from build123d import *

# Parameters (mm, degrees)
SKETCH_1_W          = 76
SKETCH_1_H          = 60
EXTRUDE_3_DEPTH     = 5.8
SKETCH_4_R          = 5.1
SKETCH_4_R_2        = 1.6
CUT_EXTRUDE_2_DEPTH = 50
FILLET_4_R          = 5
CUT_EXTRUDE_7_DEPTH = 13.5
FILLET_8_R          = 5
SKETCH_11_R         = 1
CUT_EXTRUDE_8_DEPTH = 49.76105003
SKETCH_12_R         = 1.6
CUT_EXTRUDE_9_DEPTH = 49.76105003


with BuildPart() as part:
    # ｽｹｯﾁ1 → ﾎﾞｽ - 押し出し3 (new body)
    with BuildSketch(Plane.XY):
        Rectangle(SKETCH_1_W, SKETCH_1_H)
    extrude(amount=EXTRUDE_3_DEPTH)

    # ｽｹｯﾁ4 → ｶｯﾄ - 押し出し2 (cut)
    with BuildSketch(Plane(origin=(0, 0, 0), x_dir=(-1, 0, 0), z_dir=(0, 0, -1))):
        with Locations((0, 5)):
            Circle(SKETCH_4_R)
        with Locations((-33, -5)):
            Circle(SKETCH_4_R_2)
        with Locations((-33, -25)):
            Circle(SKETCH_4_R_2)
        with Locations((33, -25)):
            Circle(SKETCH_4_R_2)
        with Locations((33, -5)):
            Circle(SKETCH_4_R_2)
    extrude(amount=-CUT_EXTRUDE_2_DEPTH, mode=Mode.SUBTRACT)

    # ﾌｨﾚｯﾄ4
    fillet_4_edges = [part.edges().sort_by_distance(p)[0] for p in [
        (38, -30, 2.9),
        (-38, -30, 2.9),
        (-38, 30, 2.9),
        (38, 30, 2.9),
    ]]
    fillet(fillet_4_edges, radius=FILLET_4_R)

    # ｽｹｯﾁ10 → ｶｯﾄ - 押し出し7 (cut)
    with BuildSketch(Plane(origin=(0, 0, 0), x_dir=(-1, 0, 0), z_dir=(0, 0, -1))):
        with BuildLine():
            Line((-38, 0), (-20, 0))
            Line((-20, 0), (-20, 5))
            ThreePointArc((-20, 5), (0, 25), (20, 5))
            Line((20, 5), (20, 0))
            Line((20, 0), (38, 0))
            Line((38, 0), (38, 30))
            Line((38, 30), (-38, 30))
            Line((-38, 30), (-38, 0))
        make_face()
    extrude(amount=-CUT_EXTRUDE_7_DEPTH, mode=Mode.SUBTRACT)

    # ﾌｨﾚｯﾄ8
    fillet_8_edges = [part.edges().sort_by_distance(p)[0] for p in [
        (-38, 0, 2.9),
        (38, 0, 2.9),
    ]]
    fillet(fillet_8_edges, radius=FILLET_8_R)

    # ｽｹｯﾁ11 → ｶｯﾄ - 押し出し8 (cut, through all)
    with BuildSketch(Plane(origin=(0, 0, 0), x_dir=(-1, 0, 0), z_dir=(0, 0, -1))):
        with Locations((-8.5, 5)):
            Circle(SKETCH_11_R)
        with Locations(Location((8.5, 5, 0), (0, 0, 180))):
            Circle(SKETCH_11_R)
    extrude(amount=-CUT_EXTRUDE_8_DEPTH, mode=Mode.SUBTRACT)

    # ｽｹｯﾁ12 → ｶｯﾄ - 押し出し9 (cut, through all)
    with BuildSketch(Plane.XY.offset(5.8)):
        with Locations((16, -20)):
            Circle(SKETCH_12_R)
    extrude(amount=-CUT_EXTRUDE_9_DEPTH, mode=Mode.SUBTRACT)


solid = part.part
Could you check a few things on this model? Use its own coordinates, in mm. A direction names the side the tool comes from. Coordinates: 2 decimals unless noted, no trailing zeros. Write each loop counter-clockwise with the first axis right and the second up, starting at its lowest first coordinate (ties: lowest second). Pieces come first, ordered by that corner, then holes. Notation, with made-up numbers: (-5.5, -17.5) - (20.5, -17.5) arc R11 ccw to (20.5, -8.5) - close; hole circle Ø6 at (39, -8). An arc over 180 degrees is marked (long way). Put each result on its own line as item: value. Start each with the question number.
Q1. Please list where these lines run through material, in increasing order: L1, parallel to Y at x = 33, z = 3.55; L2, parallel to Y at x = 23.5, z = 0.55; L3, parallel to Y at x = 0, z = 2.4.
Q2. I'm going to push flat-ended pins straight in: P1, Ø1.7, axis at x = 23.5, z = 3, coming from the +Y side; P2, Ø1.5, axis at y = 2.5, z = 2, coming from the -X side. Where does each tip first touch, or does it pass through?
Q3. Which directions (+Z, -Z, +X, -X, +Y, -Y) give clear straight access to the entire face, cutting with the end or side of a thin tool? Please do faces 1 (the flat face through (-26, 0, 3)), 2 (the flat face through (27, 0, 3)), 3 (the cylindrical face through (36, -29, 3)).
Q4. Thinking about a two-plate mould opening in Y: for faces 4 (the flat face through (0, -30, 3)), 5 (the flat face through (-1, -8, 5.8)), 6 (the cylindrical face through (9.237, 5.676, 2.859)), which applies, pulls with the +Y half, pulls with the -Y half, needs draft (parallel to the pull), parting line crosses it, or undercut?
Q5. I want a section at A-A on x = 16. Write out the boundary of the cut face in (y, z).
Q6. I want a section at D-D on x = 29. Write out the boundary of the cut face in (y, z).
Q7. I want a section at C-C on z = 2.05. Count the separate pieces of the cut face and the enclosed holes in it, plus the area to 3 significant figures.
Q8. I want a section at B-B on y = -20. Write out the boundary of the cut face in (x, z).
Checks:
1. L1: -30 to -26.6, -23.4 to -6.6, -3.4 to 0
1. L2: -30 to 0
1. L3: -30 to -0.1, 10.1 to 25
2. P1: y = 0
2. P2: x = -20
3. face 1: +Z, -Z, -X, +Y
3. face 2: +Z, -Z, +X, +Y
3. face 3: +Z, -Z, +X, -Y
4. face 4: pulls with the -Y half
4. face 5: needs draft
4. face 6: undercut
5. outline: (-30, 0) - (-21.6, 0) - (-21.6, 5.8) - (-30, 5.8) - close; (-18.4, 0) - (17, 0) - (17, 5.8) - (-18.4, 5.8) - close
6. outline: (-30, 0) - (0, 0) - (0, 5.8) - (-30, 5.8) - close
7. separate pieces: 1
7. enclosed holes: 8
7. area: 2,960 mm²
8. outline: (-38, 0) - (14.4, 0) - (14.4, 5.8) - (-38, 5.8) - close; (17.6, 0) - (38, 0) - (38, 5.8) - (17.6, 5.8) - close
